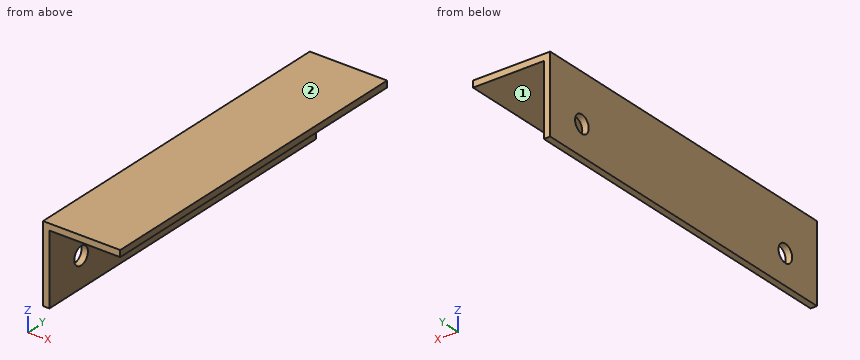
from build123d import *

# Parameters (mm, degrees)
BOSS_EXTRUDE1_DEPTH = 85.598
SKETCH2_R           = 2.1828125
CUT_EXTRUDE1_DEPTH  = 90.737520603


with BuildPart() as part:
    # Sketch1 → Boss-Extrude1 (new body)
    with BuildSketch(Plane(origin=(0, 0, 0), x_dir=(1, 0, 0), z_dir=(0, 1, 0))):
        Polygon((0, 0), (0, 19.05), (1.5875, 19.05), (1.5875, 1.5875), (19.05, 1.5875), (19.05, 0), align=None)
    extrude(amount=BOSS_EXTRUDE1_DEPTH)

    # Sketch2 → Cut-Extrude1 (cut, through all)
    with BuildSketch(Plane.ZY):
        with Locations((-11.7475, 75.438)):
            Circle(SKETCH2_R)
        with Locations((-11.7475, 10.16)):
            Circle(SKETCH2_R)
    extrude(amount=-CUT_EXTRUDE1_DEPTH, mode=Mode.SUBTRACT)


solid = part.part
Verification items for the finished model (mm, model axes). Face numbers are marked on the shaded views. A direction names the side the tool comes from. Give positions to 0.01 mm unless a question says otherwise; leave off trailing zeros. Write each loop counter-clockwise with the first axis right and the second up, starting at its lowest first coordinate (ties: lowest second). Pieces come first, ordered by that corner, then holes. Notation, with made-up numbers: M 77,-4.75 L 134,-4.75 A18 cw 134,25.25 Z; hole C -29,61 d1. An arc over 180 degrees is marked long. Use CSV: the item, a comma, the result in double quotes.
1) Material ranges on line 1 along X through (y, z) = (56.5, -7.25); line 2 along Z through (x, y) = (18, 21), recorded low to high.
Final values:
line 1,"0 to 1.59"
line 2,"-1.59 to 0"
2) Access from +Z, -Z, +X, -X, +Y, -Y to the whole of each face (thin tool, end or side, straight path). Record for the marked faces 1 and 2.
Final values:
face 1,"-Z, +X, +Y, -Y"
face 2,"+Z, +X, -X, +Y, -Y"
3) Go/stop test with flat-tipped pins: pin 1 Ø5 at (y, z) = (30.5, -5.5) entering from -X; pin 2 Ø5 at (x, y) = (7.5, 25) entering from -Z; pin 3 Ø5 at (y, z) = (34.5, -10.5) entering from +X. Record where each tip stops, or that it passes through.
Final values:
pin 1,"x = 0"
pin 2,"z = -1.59"
pin 3,"x = 1.59"
4) Cross-section at A-A (y = 10.16). Enter the section's corners in (x, z), plus the area to 3 significant figures.
Final values:
outline,"M 0,-19.05 L 1.59,-19.05 L 1.59,-13.93 L 0,-13.93 Z; M 0,-9.56 L 1.59,-9.56 L 1.59,-1.59 L 19.05,-1.59 L 19.05,0 L 0,0 Z"
area,"51.0 mm²"
5) Cross-section at C-C (z = -17). Enter the section's corners in (x, y).
Final values:
outline,"M 0,0 L 1.59,0 L 1.59,85.6 L 0,85.6 Z"
6) Cross-section at B-B (z = -12). Enter the section's corners in (x, y).
Final values:
outline,"M 0,0 L 1.59,0 L 1.59,7.99 L 0,7.99 Z; M 0,12.33 L 1.59,12.33 L 1.59,73.27 L 0,73.27 Z; M 0,77.61 L 1.59,77.61 L 1.59,85.6 L 0,85.6 Z"
7) Cross-section at D-D (y = 60). Enter the section's corners in (x, z), plus the area to 3 significant figures.
Final values:
outline,"M 0,-19.05 L 1.59,-19.05 L 1.59,-1.59 L 19.05,-1.59 L 19.05,0 L 0,0 Z"
area,"58.0 mm²"
